```python
from build123d import *

# Parameters (mm, degrees)
SKETCH1_W               = 12
SKETCH1_H               = 17
MAIN_BODY_DEPTH         = 2
SKETCH2_R               = 4
SPACER_MOUNT_DEPTH      = 5
SKETCH3_R               = 3.15
SKETCH3_R_2             = 1
BOLT_SPACER_HOLES_DEPTH = 8
FILLET1_R               = 1


with BuildPart() as part:
    # Sketch1 → main_body (new body)
    with BuildSketch(Plane(origin=(0, 0, 0), x_dir=(1, 0, 0), z_dir=(0, 1, 0))):
        with Locations((6, 8.5)):
            Rectangle(SKETCH1_W, SKETCH1_H)
    extrude(amount=MAIN_BODY_DEPTH)

    # Sketch2 → spacer_mount (add)
    with BuildSketch(Plane(origin=(0, 2, 0), x_dir=(1, 0, 0), z_dir=(0, 1, 0))):
        with Locations((6, 8.5)):
            Circle(SKETCH2_R)
    extrude(amount=SPACER_MOUNT_DEPTH)

    # Sketch3 → bolt_spacer_holes (cut, through all)
    with BuildSketch(Plane(origin=(0, 7, 0), x_dir=(1, 0, 0), z_dir=(0, 1, 0))):
        with Locations((6, 8.5)):
            Circle(SKETCH3_R)
        with Locations((6, 14.5)):
            Circle(SKETCH3_R_2)
        with Locations((6, 2.5)):
            Circle(SKETCH3_R_2)
    extrude(amount=-BOLT_SPACER_HOLES_DEPTH, mode=Mode.SUBTRACT)

    # Fillet1
    fillet1_edges = [part.edges().sort_by_distance(p)[0] for p in [
        (0, 1, -17),
        (12, 1, -17),
        (12, 1, 0),
        (0, 1, 0),
    ]]
    fillet(fillet1_edges, radius=FILLET1_R)


solid = part.part
```
Verification items for the finished model (mm, model axes). A direction names the side the tool comes from. Coordinates: 2 decimals unless noted, no trailing zeros. Loops run counter-clockwise (first coordinate to the right, second up) from the corner with the lowest first, then second, coordinate; pieces in that order, holes last. Notation, with made-up numbers: (61.5, -18) - (70.5, -18) arc R32 ccw to (70.5, 12) - close; hole circle Ø11 at (55.5, -20.75). An arc over 180 degrees is marked (long way). Return JSON: item names as keys, results as strings.
1. Section check D-D, the plane y = 6.5. Record the boundary of the cut face in (x, z), then the cut area to 3 significant figures.
Established:
{"outline": "circle Ø8 at (6, -8.5); hole circle Ø6.3 at (6, -8.5)", "area": "19.1 mm2"}
2. Section check A-A, the plane z = -2.5. Record the boundary of the cut face in (x, y), then the cut area to 3 significant figures.
Established:
{"outline": "(0, 0) - (5, 0) - (5, 2) - (0, 2) - close; (7, 0) - (12, 0) - (12, 2) - (7, 2) - close", "area": "20.0 mm2"}
3. Mould release check, pull along X, two halves, no side actions. Record for faces 3 (the cylindrical face through (5.783, 1.014, -13.524)), 4 (the flat face through (0, 1, -8)), 5 (the flat face through (4.58, 2, -12.4)): +X half, -X half, draft (parallel to the pull), parting line (faces both ways), or undercut.
Established:
{"face 3": "undercut", "face 4": "-X half", "face 5": "draft"}
4. Tool access check on faces 1 (the flat face through (12, 1, -8)), 2 (the cylindrical face through (5.133, 4.465, -4.595)). Record the directions out of +Z, -Z, +X, -X, +Y, -Y that give a thin tool (end or side, any length) a straight path to the whole face; none if there is none.
Established:
{"face 1": "+Z, -Z, +X, +Y, -Y", "face 2": "+Y"}
5. Thickness scan on L1, parallel to Z at x = 6, y = 0.8; L2, parallel to X at y = 1.55, z = -14.5; L3, parallel to Z at x = 6, y = 5.25. Record the ranges inside material, lowest first.
Established:
{"L1": "z = -17 to -15.5, -13.5 to -11.65, -5.35 to -3.5, -1.5 to 0", "L2": "x = 0 to 5, 7 to 12", "L3": "z = -12.5 to -11.65, -5.35 to -4.5"}
6. Section check C-C, the plane z = -8.5. Record the boundary of the cut face in (x, y).
Established:
{"outline": "(0, 0) - (2.85, 0) - (2.85, 7) - (2, 7) - (2, 2) - (0, 2) - close; (9.15, 0) - (12, 0) - (12, 2) - (10, 2) - (10, 7) - (9.15, 7) - close"}
7. Section check B-B, the plane x = 6. Record the boundary of the cut face in (y, z).
Established:
{"outline": "(0, -17) - (2, -17) - (2, -15.5) - (0, -15.5) - close; (0, -13.5) - (2, -13.5) - (2, -12.5) - (7, -12.5) - (7, -11.65) - (0, -11.65) - close; (0, -5.35) - (7, -5.35) - (7, -4.5) - (2, -4.5) - (2, -3.5) - (0, -3.5) - close; (0, -1.5) - (2, -1.5) - (2, 0) - (0, 0) - close"}
8. Go/stop test with flat-tipped pins: pin 1 (5 mm diameter, centred on x = 6, z = -8.5, fed in from +Y); pin 2 (1 mm diameter, centred on x = 8, y = 5, fed in from -Z); pin 3 (1 mm diameter, centred on y = 4.5, z = -6.5, fed in from +X); pin 4 (1.5 mm diameter, centred on x = 8, z = -12, fed in from +Y). Record where each tip stops, or that it passes through.
Established:
{"pin 1": "passes through", "pin 2": "stops at z = -12.21", "pin 3": "stops at x = 9.71", "pin 4": "stops at y = 7"}
